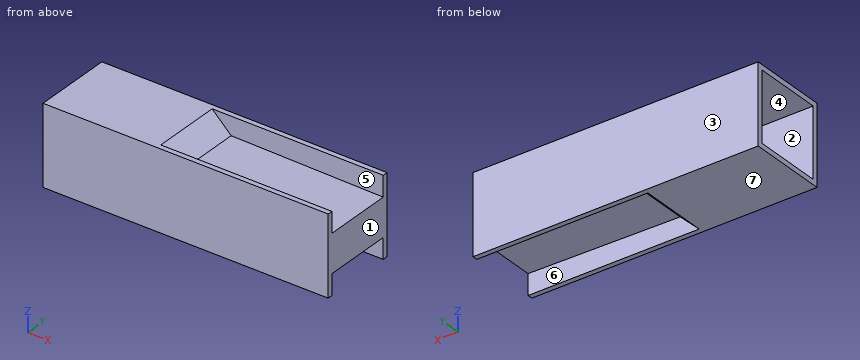
Autodesk Inventor part; units mm, degrees
ref_plane "YZ Plane" through (0, 0, 0) normal (1, 0, 0) x (0, 1, 0)
ref_plane "XZ Plane" through (0, 0, 0) normal (0, 1, 0) x (-1, 0, 0)
ref_plane "XY Plane" through (0, 0, 0) normal (0, 0, 1) x (1, 0, 0)
sketch "Sketch1" plane through (0, 0, 0) normal (0, 1, 0) x (-1, 0, 0)
  line L0 (45, 0) -> (0, 0)
  line L1 (0, 0) -> (0, -12.5)
  line L2 (0, -12.5) -> (45, -12.5)
  line L3 (45, -12.5) -> (45, 0)
  dimension "d0" = 45
  dimension "d1" = 12.5
extrude "Extrusion1" add sketch "Sketch1" along normal blind 0.8
sketch "Sketch3" plane through (0, 0, 0) normal (0, -1, 0) x (1, 0, 0)
  line L0 (-45, 0) -> (-27, 0)
  line L1 (-27, 0) -> (-24, -2.9)
  line L2 (-24, -2.9) -> (0, -3.25)
  line L3 (0, 0) -> (0, -12.5)
  line L4 (0, -9.25) -> (-24, -9.6)
  line L5 (-24, -9.6) -> (-27, -12.5)
  line L6 (0, -12.5) -> (-45, -12.5)
  line L7 (-45, -12.5) -> (-27, -12.5)
  line L8 (0, 0) -> (0, -12.5)
  line L9 (-28.7719, -3.1178) -> (-25.8887, -3.1178) construction
  line L10 (-28.7189, -9.8202) -> (-22.671, -9.5806) construction
  line L11 (-45, 0) -> (0, 0) construction
  line L12 (0, -3.25) -> (0, -9.25)
  line L13 (-45, -12.5) -> (-45, 0)
  line L14 (-45, 0) -> (-45, -0.8)
  line L15 (-45, -0.8) -> (-27.3235, -0.8)
  line L16 (-27.3235, -0.8) -> (-24.3283, -3.6953)
  line L17 (-24.3283, -3.6953) -> (-0.8, -4.0384)
  line L18 (-0.8, -4.0384) -> (-0.8, -8.4616)
  line L19 (-0.8, -8.4616) -> (-24.3283, -8.8047)
  line L20 (-24.3283, -8.8047) -> (-27.3235, -11.7)
  line L21 (-27.3235, -11.7) -> (-45, -11.7)
  line L22 (-45, -12.5) -> (-45, -11.7)
  dimension "d6" = 18
  dimension "d7" = 6.7
  dimension "d9" = 2.9
  dimension "d10" = 6
  dimension "d12" = 24
  dimension "d13" = 3.25
  dimension "d14" = 0.8
  dimension "d15" = 0.8
  dimension "d16" = 0.8
  dimension "d17" = 0.8
  dimension "d18" = 0.8
  dimension "d19" = 0.8
  dimension "d20" = 0.8
extrude "Extrusion2" add sketch "Sketch3" along normal blind 10.9 contours L0 L1 L2 L3 L4 L5 L6 L13 L21 L20 L19 L18 L17 L16 L15
sketch "Sketch4" plane through (0, -10.9, 0) normal (0, -1, 0) x (1, 0, 0)
  line L0 (0, 0) -> (0, -12.5)
  line L1 (-45, 0) -> (0, 0)
  line L2 (0, 0) -> (0, -12.5)
  line L3 (0, -12.5) -> (-45, -12.5)
  line L4 (-45, -12.5) -> (-45, 0)
extrude "Extrusion3" add sketch "Sketch4" along normal blind 0.8
properties part number "Cuvette" material "Polycarbonate, Clear"
Source: CAD feature listing. Evaluate the final solid. Frame: model axes, mm. Face numbers are marked on the shaded views. A direction names the side the tool comes from. Round coordinates to 2 decimals unless told otherwise and drop trailing zeros. Loops run counter-clockwise (first coordinate to the right, second up) from the corner with the lowest first, then second, coordinate; pieces in that order, holes last. Notation, with made-up numbers: M -2,86.5 L 2,86.5 A30 cw 2,113.5 Z; hole C 4.5,64 d10. An arc over 180 degrees is marked long. Put each result on its own line as item: value.
(1) Section C-C, the plane z = -6.5. Return loops of the section in (x, y).
Solutions:
outline: M -45,-11.7 L 0,-11.7 L 0,0.8 L -45,0.8 L -45,0 L -0.8,0 L -0.8,-10.9 L -45,-10.9 Z
(2) First-contact query: pin 1 (5 mm diameter, centred on y = -7, z = -7, fed in from -X); pin 2 (1.5 mm diameter, centred on x = -15, y = -9.5, fed in from +Z). Flat tips, straight axial feed; report the tip coordinate or a pass-through.
Solutions:
pin 1: x = -25.05
pin 2: z = -3.02
(3) Pull-direction query (X, two-part tool) for the marked faces 1 and 2; classes: released by +X, released by -X, zero draft, split by the parting line, or undercut.
Solutions:
face 1: released by +X
face 2: zero draft
(4) Ray query, line 1 (Z direction, x = -28, y = -2.5); line 2 (Y direction, x = -36.5, z = -6); line 3 (X direction, y = -8, z = -6.75). Return the intervals inside material, ascending. Write a range as [from, to].
Solutions:
line 1: [-12.5, -11.7], [-0.8, 0]
line 2: [-11.7, -10.9], [0, 0.8]
line 3: [-0.8, 0]
(5) Access query for the marked faces 3, 4, 5, 6 and 7. Directions: +Z, -Z, +X, -X, +Y, -Y. A direction counts if a zero-diameter tool reaches every point of the face in a straight line with its end or side. Return the directions, or none.
Solutions:
face 3: +Z, -Z, +X, -X, +Y
face 4: -X
face 5: +Z, +X
face 6: -Z, +X
face 7: -Z, +X, -X, +Y, -Y
(6) Section D-D, the plane x = -21.5. Return loops of the section in (y, z).
Solutions:
outline: M -11.7,-12.5 L -10.9,-12.5 L -10.9,-9.56 L 0,-9.56 L 0,-12.5 L 0.8,-12.5 L 0.8,0 L 0,0 L 0,-2.94 L -10.9,-2.94 L -10.9,0 L -11.7,0 Z; hole M -10.9,-8.76 L 0,-8.76 L 0,-3.74 L -10.9,-3.74 Z
(7) Section B-B, the plane y = -0.5. Return loops of the section in (x, z), and give its area (3 significant figures).
Solutions:
outline: M -45,-12.5 L -27,-12.5 L -24,-9.6 L 0,-9.25 L 0,-3.25 L -24,-2.9 L -27,0 L -45,0 L -45,-0.8 L -27.32,-0.8 L -24.33,-3.7 L -0.8,-4.04 L -0.8,-8.46 L -24.33,-8.8 L -27.32,-11.7 L -45,-11.7 Z
area: 77.4 mm²
(8) Section A-A, the plane x = -41. Return loops of the section in (y, z).
Solutions:
outline: M -11.7,-12.5 L 0.8,-12.5 L 0.8,0 L -11.7,0 Z; hole M -10.9,-11.7 L 0,-11.7 L 0,-0.8 L -10.9,-0.8 Z
